Part print with two shaded views. Sizes in mm from the minimum x, y, z corner. A direction names the side the tool comes from. Round coordinates to 2 decimals unless told otherwise and drop trailing zeros. Loops run counter-clockwise (first coordinate to the right, second up) from the corner with the lowest first, then second, coordinate; pieces in that order, holes last. Notation, with made-up numbers: M 36.25,28 L 52.25,28 A23 ccw 52.25,42 Z; hole C -21.75,-6 d8. An arc over 180 degrees is marked long. Use a Markdown table: item, result. Add a question column.
Item 1: Saw through at A-A on z = 17.5. Write the cut outline in (x, y).
Item 2: Saw through at B-B on y = 4.5. Write the cut outline in (x, z), then the cut area to 3 significant figures.
Item 3: Pin check, flat tips, straight feed: P1, Ø10, axis at y = 9.5, z = 5, coming from the -X side; P2, Ø10, axis at y = 11, z = 15.5, coming from the +X side; P3, Ø7.5, axis at x = 2.5, z = 5.5, coming from the +Y side. Stop position of each tip, or through.
Item 4: Wall check: L1, parallel to X at y = 14.5, z = 13; L2, parallel to Y at x = 3.5, z = 17. Give the ranges that are in metal, low to high. Write a range as from..to.
Item 5: Tool access for the marked faces 1, 2 and 3: list every direction of +Z, -Z, +X, -X, +Y, -Y with a clear straight run to the whole face (end or side of a thin tool).
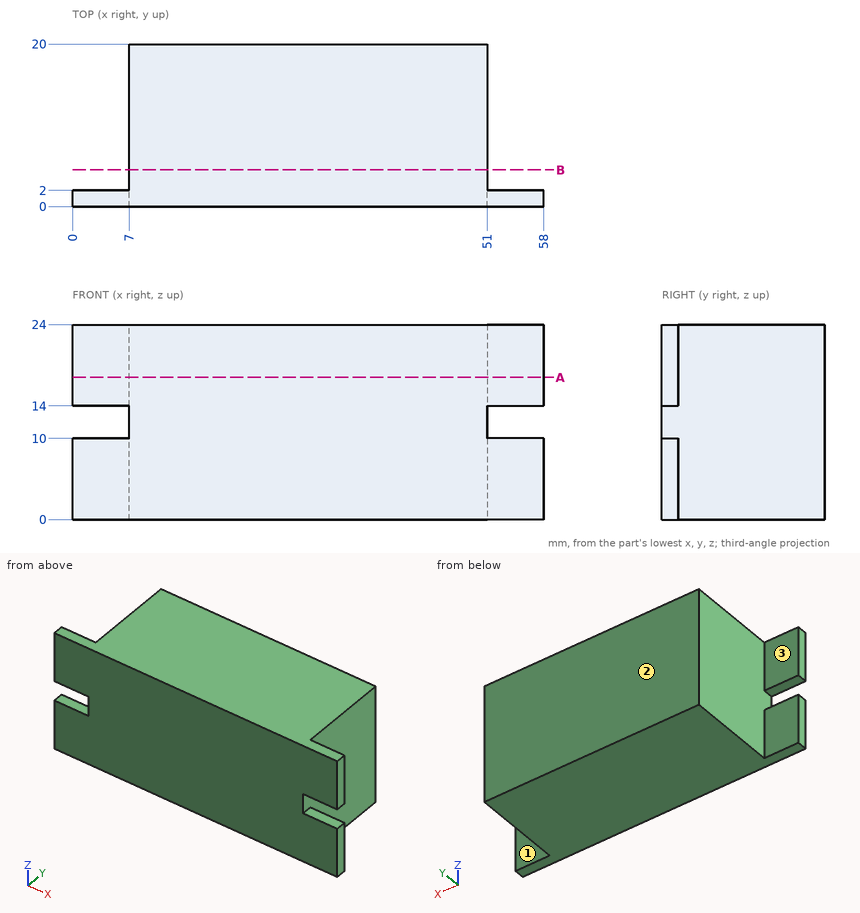
Entries:
| question | item | result |
|---|---|---|
| 1 | outline | M 0,0 L 58,0 L 58,2 L 51,2 L 51,20 L 7,20 L 7,2 L 0,2 Z |
| 2 | outline | M 7,0 L 51,0 L 51,24 L 7,24 Z |
| 2 | area | 1,060 mm2 |
| 3 | P1 | x = 7 |
| 3 | P2 | x = 51 |
| 3 | P3 | y = 2 |
| 4 | L1 | 7..51 |
| 4 | L2 | 0..2 |
| 5 | face 1 | +Z, -Z, +X, +Y |
| 5 | face 2 | +Z, -Z, +X, -X, +Y |
| 5 | face 3 | +Z, -Z, -X, +Y |
